from build123d import *

# Parameters (mm, degrees)
BOSS_EXTRUDE1_DEPTH     = 27
BOSS_EXTRUDE2_START     = -2
BOSS_EXTRUDE2_DEPTH     = 2
BOSS_EXTRUDE3_DEPTH     = 4
BOSS_EXTRUDE4_DEPTH     = 2
CUT_EXTRUDE1_DEPTH      = 49.441415403
CUT_EXTRUDE1_DEPTH_BACK = 49.441415403
BOSS_EXTRUDE8_DEPTH     = 2
BOSS_EXTRUDE9_DEPTH     = 4
CUT_EXTRUDE2_DEPTH      = 49.441415403
CUT_EXTRUDE2_DEPTH_BACK = 49.441415403
SKETCH5_R               = 4


# Read off the part's stored shape, not the designer's step: Boss-Extrude2
with BuildPart() as part:
    # Sketch2 → Boss-Extrude1 (new body)
    with BuildSketch(Plane(origin=(0, 0, 0), x_dir=(1, 0, 0), z_dir=(0, 1, 0))):
        Polygon((22.563885141, -12.154202836), (25.497523714, -2.594194221), (24.549395438, 7.360756948), (19.863844247, 16.195099597), (12.154202836, 22.563885141), (2.594194221, 25.497523714), (-7.360756948, 24.549395438), (-16.195099597, 19.863844247), (-22.563885141, 12.154202836), (-25.497523714, 2.594194221), (-24.549395438, -7.360756948), (-19.863844247, -16.195099597), (-12.154202836, -22.563885141), (-2.594194221, -25.497523714), (7.360756948, -24.549395438), (16.195099597, -19.863844247), align=None)
    extrude(amount=BOSS_EXTRUDE1_DEPTH)



with BuildPart() as body_2:
    # Boss-Extrude2 outline → Boss-Extrude2 (new body)
    with BuildSketch(Plane(origin=(0, 27, 0), x_dir=(1, 0, 0), z_dir=(0, 1, 0)).offset(BOSS_EXTRUDE2_START)):
        Polygon((-8.20996139, 27.38163889), (-18.063514845, 22.155519532), (-25.167061911, 13.556423167), (-28.439151941, 2.893484263), (-27.38163889, -8.20996139), (-22.155519532, -18.063514845), (-13.556423167, -25.167061911), (-2.893484263, -28.439151941), (8.20996139, -27.38163889), (18.063514845, -22.155519532), (25.167061911, -13.556423167), (28.439151941, -2.893484263), (27.38163889, 8.20996139), (22.155519532, 18.063514845), (13.556423167, 25.167061911), (2.893484263, 28.439151941), align=None)
        Polygon((-12.154202836, -22.563885141), (-13.045832812, -23.643234938), (-20.755474224, -17.274449394), (-19.863844247, -16.195099597), align=None, mode=Mode.SUBTRACT)
        Polygon((-24.549395438, -7.360756948), (-25.943088602, -7.493494906), (-26.891216878, 2.461456262), (-25.497523714, 2.594194221), align=None, mode=Mode.SUBTRACT)
        Polygon((7.360756948, -24.549395438), (7.493494906, -25.943088602), (-2.461456262, -26.891216878), (-2.594194221, -25.497523714), align=None, mode=Mode.SUBTRACT)
        Polygon((17.274449394, -20.755474224), (16.195099597, -19.863844247), (22.563885141, -12.154202836), (23.643234938, -13.045832812), align=None, mode=Mode.SUBTRACT)
        Polygon((-22.563885141, 12.154202836), (-23.643234938, 13.045832812), (-17.274449394, 20.755474224), (-16.195099597, 19.863844247), align=None, mode=Mode.SUBTRACT)
        Polygon((-7.493494906, 25.943088602), (2.461456262, 26.891216878), (2.594194221, 25.497523714), (-7.360756948, 24.549395438), align=None, mode=Mode.SUBTRACT)
        Polygon((26.891216878, -2.461456262), (25.497523714, -2.594194221), (24.549395438, 7.360756948), (25.943088602, 7.493494906), align=None, mode=Mode.SUBTRACT)
        Polygon((20.755474224, 17.274449394), (19.863844247, 16.195099597), (12.154202836, 22.563885141), (13.045832812, 23.643234938), align=None, mode=Mode.SUBTRACT)
    extrude(amount=BOSS_EXTRUDE2_DEPTH)


with BuildPart() as body_3:
    # Sketch4 → Boss-Extrude3 (new body)
    with BuildSketch(Plane(origin=(0, 0, 0), x_dir=(-1, 0, 0), z_dir=(0, -1, 0))):
        Polygon((18.063514845, 22.155519532), (8.20996139, 27.38163889), (-2.893484263, 28.439151941), (-13.556423167, 25.167061911), (-22.155519532, 18.063514845), (-27.38163889, 8.20996139), (-28.439151941, -2.893484263), (-25.167061911, -13.556423167), (-18.063514845, -22.155519532), (-8.20996139, -27.38163889), (2.893484263, -28.439151941), (13.556423167, -25.167061911), (22.155519532, -18.063514845), (27.38163889, -8.20996139), (28.439151941, 2.893484263), (25.167061911, 13.556423167), align=None)
        Polygon((-2.738679069, 26.9176201), (-12.831136789, 23.820591168), (-20.970170247, 17.097093165), (-25.91668538, 7.770717713), (-26.9176201, -2.738679069), (-23.820591168, -12.831136789), (-17.097093165, -20.970170247), (-7.770717713, -25.91668538), (2.738679069, -26.9176201), (12.831136789, -23.820591168), (20.970170247, -17.097093165), (25.91668538, -7.770717713), (26.9176201, 2.738679069), (23.820591168, 12.831136789), (17.097093165, 20.970170247), (7.770717713, 25.91668538), align=None, mode=Mode.SUBTRACT)
    extrude(amount=-BOSS_EXTRUDE3_DEPTH)


with BuildPart() as part_1:
    add(part.part)

    add(body_3.part)  # Boss-Extrude4 merges body 3
    # Sketch4_4 → Boss-Extrude4 (add)
    with BuildSketch(Plane(origin=(0, 0, 0), x_dir=(-1, 0, 0), z_dir=(0, -1, 0))):
        Polygon((7.770717713, 25.91668538), (-2.738679069, 26.9176201), (-12.831136789, 23.820591168), (-20.970170247, 17.097093165), (-25.91668538, 7.770717713), (-26.9176201, -2.738679069), (-23.820591168, -12.831136789), (-17.097093165, -20.970170247), (-7.770717713, -25.91668538), (2.738679069, -26.9176201), (12.831136789, -23.820591168), (20.970170247, -17.097093165), (25.91668538, -7.770717713), (26.9176201, 2.738679069), (23.820591168, 12.831136789), (17.097093165, 20.970170247), align=None)
        Polygon((24.549395438, -7.360756948), (25.497523714, 2.594194221), (22.563885141, 12.154202836), (16.195099597, 19.863844247), (7.360756948, 24.549395438), (-2.594194221, 25.497523714), (-12.154202836, 22.563885141), (-19.863844247, 16.195099597), (-24.549395438, 7.360756948), (-25.497523714, -2.594194221), (-22.563885141, -12.154202836), (-16.195099597, -19.863844247), (-7.360756948, -24.549395438), (2.594194221, -25.497523714), (12.154202836, -22.563885141), (19.863844247, -16.195099597), align=None, mode=Mode.SUBTRACT)
    extrude(amount=-BOSS_EXTRUDE4_DEPTH)


with BuildPart() as cut_extrude1_tool:
    # Sketch3_3 → Cut-Extrude1 (new, two sides: drawn at the far end of the back side and taken through both)
    with BuildSketch(Plane(origin=(0, 27, 0), x_dir=(1, 0, 0), z_dir=(0, 1, 0)).offset(-CUT_EXTRUDE1_DEPTH_BACK)):
        Polygon((-25.497523714, 2.594194221), (-22.563885141, 12.154202836), (-23.902286347, 12.564912236), (-26.835924921, 3.004903621), align=None)
        Polygon((-16.195099597, 19.863844247), (-7.360756948, 24.549395438), (-8.016734114, 25.786203409), (-16.851076763, 21.100652218), align=None)
        Polygon((3.004903621, 26.835924921), (2.594194221, 25.497523714), (12.154202836, 22.563885141), (12.564912236, 23.902286347), align=None)
        Polygon((21.100652218, 16.851076763), (19.863844247, 16.195099597), (24.549395438, 7.360756948), (25.786203409, 8.016734114), align=None)
        Polygon((26.835924921, -3.004903621), (25.497523714, -2.594194221), (22.563885141, -12.154202836), (23.902286347, -12.564912236), align=None)
        Polygon((16.851076763, -21.100652218), (16.195099597, -19.863844247), (7.360756948, -24.549395438), (8.016734114, -25.786203409), align=None)
        Polygon((-2.594194221, -25.497523714), (-12.154202836, -22.563885141), (-12.564912236, -23.902286347), (-3.004903621, -26.835924921), align=None)
        Polygon((-19.863844247, -16.195099597), (-24.549395438, -7.360756948), (-25.786203409, -8.016734114), (-21.100652218, -16.851076763), align=None)
    extrude(amount=CUT_EXTRUDE1_DEPTH + CUT_EXTRUDE1_DEPTH_BACK)


with BuildPart() as part_2:
    add(part_1.part)

    # Cut-Extrude1: cut by cut_extrude1_tool
    add(cut_extrude1_tool.part, mode=Mode.SUBTRACT)



with BuildPart() as body_2_1:
    add(body_2.part)

    # Cut-Extrude1: cut by cut_extrude1_tool
    add(cut_extrude1_tool.part, mode=Mode.SUBTRACT)


with BuildPart() as part_3:
    add(part_2.part)

    add(body_2_1.part)  # Boss-Extrude8 merges body 2
    # Sketch3_5 → Boss-Extrude8 (add)
    with BuildSketch(Plane(origin=(0, 27, 0), x_dir=(1, 0, 0), z_dir=(0, 1, 0))):
        Polygon((-16.195099597, 19.863844247), (-7.360756948, 24.549395438), (-8.016734114, 25.786203409), (-16.851076763, 21.100652218), align=None)
        Polygon((3.004903621, 26.835924921), (2.594194221, 25.497523714), (12.154202836, 22.563885141), (12.564912236, 23.902286347), align=None)
        Polygon((-25.497523714, 2.594194221), (-22.563885141, 12.154202836), (-23.902286347, 12.564912236), (-26.835924921, 3.004903621), align=None)
        Polygon((21.100652218, 16.851076763), (19.863844247, 16.195099597), (24.549395438, 7.360756948), (25.786203409, 8.016734114), align=None)
        Polygon((-19.863844247, -16.195099597), (-24.549395438, -7.360756948), (-25.786203409, -8.016734114), (-21.100652218, -16.851076763), align=None)
        Polygon((26.835924921, -3.004903621), (25.497523714, -2.594194221), (22.563885141, -12.154202836), (23.902286347, -12.564912236), align=None)
        Polygon((-2.594194221, -25.497523714), (-12.154202836, -22.563885141), (-12.564912236, -23.902286347), (-3.004903621, -26.835924921), align=None)
        Polygon((16.851076763, -21.100652218), (16.195099597, -19.863844247), (7.360756948, -24.549395438), (8.016734114, -25.786203409), align=None)
    extrude(amount=-BOSS_EXTRUDE8_DEPTH)

    # Sketch3_6 → Boss-Extrude9 (add)
    with BuildSketch(Plane(origin=(0, 27, 0), x_dir=(1, 0, 0), z_dir=(0, 1, 0))):
        Polygon((2.893484263, 28.439151941), (-8.20996139, 27.38163889), (-18.063514845, 22.155519532), (-25.167061911, 13.556423167), (-28.439151941, 2.893484263), (-27.38163889, -8.20996139), (-22.155519532, -18.063514845), (-13.556423167, -25.167061911), (-2.893484263, -28.439151941), (8.20996139, -27.38163889), (18.063514845, -22.155519532), (25.167061911, -13.556423167), (28.439151941, -2.893484263), (27.38163889, 8.20996139), (22.155519532, 18.063514845), (13.556423167, 25.167061911), align=None)
        Polygon((-7.770717713, 25.91668538), (-7.493494906, 25.943088602), (-4.248833717, 26.252116237), (2.461456262, 26.891216878), (2.738679069, 26.9176201), (3.004903621, 26.835924921), (12.564912236, 23.902286347), (12.831136789, 23.820591168), (13.045832812, 23.643234938), (20.755474224, 17.274449394), (20.970170247, 17.097093165), (21.100652218, 16.851076763), (25.786203409, 8.016734114), (25.91668538, 7.770717713), (25.943088602, 7.493494906), (26.891216878, -2.461456262), (26.9176201, -2.738679069), (26.835924921, -3.004903621), (23.902286347, -12.564912236), (23.820591168, -12.831136789), (23.643234938, -13.045832812), (17.274449394, -20.755474224), (17.097093165, -20.970170247), (16.851076763, -21.100652218), (8.016734114, -25.786203409), (7.770717713, -25.91668538), (7.493494906, -25.943088602), (-2.461456262, -26.891216878), (-2.738679069, -26.9176201), (-3.004903621, -26.835924921), (-12.564912236, -23.902286347), (-12.831136789, -23.820591168), (-13.045832812, -23.643234938), (-20.755474224, -17.274449394), (-20.970170247, -17.097093165), (-21.100652218, -16.851076763), (-25.786203409, -8.016734114), (-25.91668538, -7.770717713), (-25.943088602, -7.493494906), (-26.891216878, 2.461456262), (-26.9176201, 2.738679069), (-26.835924921, 3.004903621), (-23.902286347, 12.564912236), (-23.820591168, 12.831136789), (-23.643234938, 13.045832812), (-17.274449394, 20.755474224), (-17.097093165, 20.970170247), (-16.851076763, 21.100652218), (-8.016734114, 25.786203409), align=None, mode=Mode.SUBTRACT)
    extrude(amount=-BOSS_EXTRUDE9_DEPTH)

    # Sketch5 → Cut-Extrude2 (cut, two sides: drawn at the far end of the back side and taken through both)
    with BuildSketch(Plane.XZ.offset(-CUT_EXTRUDE2_DEPTH_BACK)):
        with Locations(Location((0, 0, 0), (0, 0, 270))):
            Circle(SKETCH5_R)
    extrude(amount=CUT_EXTRUDE2_DEPTH + CUT_EXTRUDE2_DEPTH_BACK, mode=Mode.SUBTRACT)


solid = part_3.part
For this review, take the finished solid that the model builds, in its own axes (mm). A direction names the side the tool comes from. Round coordinates to 2 decimals unless told otherwise and drop trailing zeros. Order: outer loops, then holes, each group sorted by start corner. A loop starts at its lowest first (then second) coordinate and runs counter-clockwise, first axis right, second up. Notation, with made-up numbers: (15, -24) -> (49, -24) arc R14 ccw to (49, 3) -> close; hole circle Ø2 at (10, 4.5). An arc over 180 degrees is marked (long way). Put each result on its own line as item: value.
Q1. Insertion check: pin 1 Ø4 at (x, y) = (-4, 4.5) entering from -Z; pin 2 Ø5 at (x, z) = (0, 0) entering from +Y; pin 3 Ø1.5 at (x, y) = (11, 20) entering from -Z; pin 4 Ø1.5 at (x, y) = (-9, 8) entering from +Z. Each pin has a flat end and moves straight along its axis. Give the tip position at first contact, or say it passes through.
Check result:
pin 1: z = -27.97
pin 2: through
pin 3: z = -23.15
pin 4: z = 23.76
Q2. For probe 1 along Z at (x, y) = (7.5, 3); probe 2 along Z at (x, y) = (-22, 4.5); probe 3 along Y at (x, z) = (-15, -22), list the stretches that pass through material, from the lowest coordinate up. Write a range as [from, to].
Check result:
probe 1: [-27.03, -25.46], [-23.99, 24.48], [25.94, 27.45]
probe 2: [-12.84, 12.17]
probe 3: [25, 27]
Q3. Mouldability with a two-part tool opening along Z and no side actions: class faces 4 (the flat face through (3, 2, 26)), 5 (the flat face through (27.903, 1.972, -2.736)), 6 (the flat face through (-17.796, 1.972, 21.665)) as pulls with the +Z half, pulls with the -Z half, needs draft (parallel to the pull), parting line crosses it, or undercut.
Check result:
face 4: undercut
face 5: pulls with the -Z half
face 6: pulls with the +Z half
Q4. Add section D-D on x = 0. Write out the cut boundary in (y, z), plus the area to 3 significant figures.
Check result:
outline: (0, -28.16) -> (4, -28.16) -> (4, -26.66) -> (2, -26.66) -> (2, -25.25) -> (27, -25.25) -> (27, -4) -> (0, -4) -> close; (0, 4) -> (27, 4) -> (27, 25.25) -> (2, 25.25) -> (2, 26.66) -> (4, 26.66) -> (4, 28.16) -> (0, 28.16) -> close; (23, -28.16) -> (27, -28.16) -> (27, -26.66) -> (23, -26.66) -> close; (23, 26.66) -> (27, 26.66) -> (27, 28.16) -> (23, 28.16) -> close
area: 1,180 mm2
Q5. Add section A-A on z = 0. Write out the cut boundary in (x, y).
Check result:
outline: (-28.16, 0) -> (-4, 0) -> (-4, 27) -> (-25.25, 27) -> (-25.25, 2) -> (-26.66, 2) -> (-26.66, 4) -> (-28.16, 4) -> close; (-28.16, 23) -> (-26.66, 23) -> (-26.66, 27) -> (-28.16, 27) -> close; (4, 0) -> (28.16, 0) -> (28.16, 4) -> (26.66, 4) -> (26.66, 2) -> (25.25, 2) -> (25.25, 27) -> (4, 27) -> close; (26.66, 23) -> (28.16, 23) -> (28.16, 27) -> (26.66, 27) -> close
Q6. Machinability: for faces 1 (the flat face through (-24.805, 25.028, 13.068)), 2 (the flat face through (-24.05, 12.32, -7.31)), 3 (the flat face through (25.03, 14.32, -2.31)), which of the approach directions +Z, -Z, +X, -X, +Y, -Y give a long, thin tool a straight path to every point of the face, cutting with its end or side? Answer none if there is none.
Check result:
face 1: +Z, -X, +Y, -Y
face 2: -Y
face 3: +Y
Q7. Add section B-B on y = 12.75. Write out the cut boundary in (x, z).
Check result:
outline: (-25.5, -2.59) -> (-22.56, -12.15) -> (-16.2, -19.86) -> (-7.36, -24.55) -> (2.59, -25.5) -> (12.15, -22.56) -> (19.86, -16.2) -> (24.55, -7.36) -> (25.5, 2.59) -> (22.56, 12.15) -> (16.2, 19.86) -> (7.36, 24.55) -> (-2.59, 25.5) -> (-12.15, 22.56) -> (-19.86, 16.2) -> (-24.55, 7.36) -> close; hole circle Ø8 at (0, 0)
Q8. Add section C-C on x = 19. Write out the cut boundary in (y, z).
Check result:
outline: (0, -20.67) -> (4, -20.67) -> (4, -18.72) -> (2, -18.72) -> (2, -16.91) -> (27, -16.91) -> (27, 16.47) -> (2, 16.47) -> (2, 18.67) -> (4, 18.67) -> (4, 21.02) -> (0, 21.02) -> close; (23, -20.67) -> (27, -20.67) -> (27, -18.72) -> (23, -18.72) -> close; (23, 18.67) -> (27, 18.67) -> (27, 21.02) -> (23, 21.02) -> close
